Build history of the part. All positions in model axes, mm. A direction names the side the tool comes from. Coordinates: 2 decimals unless noted, no trailing zeros. Write each loop counter-clockwise with the first axis right and the second up, starting at its lowest first coordinate (ties: lowest second). Pieces come first, ordered by that corner, then holes.
from build123d import *

# Parameters (mm, degrees)
SKETCH1_R           = 1.5
BOSS_EXTRUDE1_DEPTH = 2
SKETCH2_W           = 30.25
SKETCH2_H           = 7
BOSS_EXTRUDE2_DEPTH = 10
CUT_EXTRUDE1_DEPTH  = 72.688562547
SKETCH4_W           = 15
SKETCH4_H           = 18.5
BOSS_EXTRUDE3_DEPTH = 15
SKETCH5_W           = 6.5
SKETCH5_H           = 4
BOSS_EXTRUDE4_DEPTH = 4
SKETCH6_R           = 1.5
BOSS_EXTRUDE5_DEPTH = 5
FILLET1_R           = 1.5
FILLET2_R           = 1.5
FILLET3_R           = 1.5
FILLET4_R           = 1.5
FILLET5_R           = 1.5


with BuildPart() as part:
    # Sketch1 → Boss-Extrude1 (new body)
    with BuildSketch(Plane(origin=(0, 0, 0), x_dir=(1, 0, 0), z_dir=(0, 1, 0))):
        with BuildLine():
            Line((-35, -22.5), (35, -22.5))
            ThreePointArc((35, -22.5), (35.707106781, -22.207106781), (36, -21.5))
            Line((36, -21.5), (36, 21.5))
            ThreePointArc((36, 21.5), (35.707106781, 22.207106781), (35, 22.5))
            Line((35, 22.5), (-35, 22.5))
            ThreePointArc((-35, 22.5), (-35.707106781, 22.207106781), (-36, 21.5))
            Line((-36, 21.5), (-36, -21.5))
            ThreePointArc((-36, -21.5), (-35.707106781, -22.207106781), (-35, -22.5))
        make_face()
        with Locations(Location((-33.5, 20, 0), (0, 0, 270))):
            Circle(SKETCH1_R, mode=Mode.SUBTRACT)
        with Locations(Location((33.5, 20, 0), (0, 0, 90))):
            Circle(SKETCH1_R, mode=Mode.SUBTRACT)
        with Locations(Location((33.5, -20, 0), (0, 0, 270))):
            Circle(SKETCH1_R, mode=Mode.SUBTRACT)
        with Locations(Location((-33.5, -20, 0), (0, 0, 90))):
            Circle(SKETCH1_R, mode=Mode.SUBTRACT)
    extrude(amount=BOSS_EXTRUDE1_DEPTH)

    # Sketch2 → Boss-Extrude2 (add)
    with BuildSketch(Plane(origin=(0, 2, 0), x_dir=(1, 0, 0), z_dir=(0, 1, 0))):
        with Locations((-15.875, 16)):
            Rectangle(SKETCH2_W, SKETCH2_H)
        with Locations((15.875, 16)):
            Rectangle(SKETCH2_W, SKETCH2_H)
    extrude(amount=BOSS_EXTRUDE2_DEPTH)

    # Sketch3 → Cut-Extrude1 (cut, through all)
    with BuildSketch(Plane.ZY.offset(31)):
        Polygon((-19.5, 8), (-18.5, 12), (-19.5, 12), align=None)
        Polygon((-12.5, 8), (-14, 12), (-12.5, 12), align=None)
    extrude(amount=-CUT_EXTRUDE1_DEPTH, mode=Mode.SUBTRACT)

    # Sketch4 → Boss-Extrude3 (add)
    with BuildSketch(Plane(origin=(0, 2, 0), x_dir=(1, 0, 0), z_dir=(0, 1, 0))):
        with Locations((26, 2.25)):
            Rectangle(SKETCH4_W, SKETCH4_H)
        with Locations((8.5, 2.25)):
            Rectangle(SKETCH4_W, SKETCH4_H)
        with Locations((-8.5, 2.25)):
            Rectangle(SKETCH4_W, SKETCH4_H)
        with Locations((-26, 2.25)):
            Rectangle(SKETCH4_W, SKETCH4_H)
    extrude(amount=BOSS_EXTRUDE3_DEPTH)

    # Sketch5 → Boss-Extrude4 (add)
    with BuildSketch(Plane(origin=(0, 2, 0), x_dir=(1, 0, 0), z_dir=(0, 1, 0))):
        with Locations((-26, -10.5)):
            Rectangle(SKETCH5_W, SKETCH5_H)
        with Locations((-8.5, -10.5)):
            Rectangle(SKETCH5_W, SKETCH5_H)
        with Locations((8.5, -10.5)):
            Rectangle(SKETCH5_W, SKETCH5_H)
        with Locations((26, -10.5)):
            Rectangle(SKETCH5_W, SKETCH5_H)
    extrude(amount=BOSS_EXTRUDE4_DEPTH)

    # Sketch6 → Boss-Extrude5 (add)
    with BuildSketch(Plane(origin=(0, 2, 0), x_dir=(1, 0, 0), z_dir=(0, 1, 0))):
        with Locations(Location((28, -19, 0), (0, 0, 90))):
            Circle(SKETCH6_R)
        with Locations(Location((21.5, -19, 0), (0, 0, 90))):
            Circle(SKETCH6_R)
        with Locations(Location((15, -19, 0), (0, 0, 90))):
            Circle(SKETCH6_R)
        with Locations(Location((8.5, -19, 0), (0, 0, 90))):
            Circle(SKETCH6_R)
        with Locations(Location((2, -19, 0), (0, 0, 90))):
            Circle(SKETCH6_R)
    extrude(amount=BOSS_EXTRUDE5_DEPTH)

    # Fillet1
    fillet1_edges = [part.edges().sort_by_distance(p)[0] for p in [
        (2, 7, 20.5),
    ]]
    fillet(fillet1_edges, radius=FILLET1_R)

    # Fillet2
    fillet2_edges = [part.edges().sort_by_distance(p)[0] for p in [
        (8.5, 7, 20.5),
    ]]
    fillet(fillet2_edges, radius=FILLET2_R)

    # Fillet3
    fillet3_edges = [part.edges().sort_by_distance(p)[0] for p in [
        (15, 7, 20.5),
    ]]
    fillet(fillet3_edges, radius=FILLET3_R)

    # Fillet4
    fillet4_edges = [part.edges().sort_by_distance(p)[0] for p in [
        (21.5, 7, 20.5),
    ]]
    fillet(fillet4_edges, radius=FILLET4_R)

    # Fillet5
    fillet5_edges = [part.edges().sort_by_distance(p)[0] for p in [
        (28, 7, 20.5),
    ]]
    fillet(fillet5_edges, radius=FILLET5_R)


solid = part.part
(1) Probe L1, parallel to X at y = 2.75, z = -6; L2, parallel to X at y = 0.65, z = 20; L3, parallel to Z at x = 5, y = 4.75. List the from-to ranges inside material, lowest first.
(2) Slice it at A-A, the plane x = 25. List the corners of the cut face in (y, z), and give its area (4 significant figures).
(3) Slice it at C-C, the plane z = -10. List the corners of the cut face in (x, y), and give its area (3 significant figures).
(4) 3-axis set-ups, long thin cutter, end or side, ignore diameter. For faces 4 (the flat face through (26, 9, 7)), 5 (the flat face through (-9, 6, 10)), 6 (the cylindrical face through (14.93, 3.73, 20.5)): which of +Z, -Z, +X, -X, +Y, -Y reach the whole face in a straight line?
(5) Slice it at D-D, the plane y = 4.5. Give the number of separate pieces and of enclosed holes in the cut face, and give its area (3 significant figures).
(6) Slice it at B-B, the plane y = 9. List the corners of the cut face in (x, z) (3 decimals), and give its area (3 significant figures).
(7) Flat gauge pins, fed straight in: P1, Ø6.5, axis at x = -13, y = 6.5, coming from the -Z side; P2, Ø1, axis at x = -28.5, y = 7.5, coming from the +Z side; P3, Ø5, axis at x = -15, z = -17, coming from the +Y side. Where does each tip first touch, or does it go through?
(8) Two-plate mould, pull along X, no slides. Class faces 1 (the flat face through (8, 4, 8.5)), 2 (the flat face through (18.5, 9, -2)), 3 (the flat face through (-33.5, 9, -2)): pulls with the +X half, pulls with the -X half, needs draft (parallel to the pull), parting line crosses it, or undercut.
Results:
1. L1: x = -33.5 to -18.5, -16 to -1, 1 to 16, 18.5 to 33.5
1. L2: x = -36 to -35, -32 to 32, 35 to 36
1. L3: z = -19.5 to -12.5, -11.5 to 7
2. outline: (0, -22.5) - (2, -22.5) - (2, -19.5) - (8, -19.5) - (12, -18.5) - (12, -14) - (8, -12.5) - (2, -12.5) - (2, -11.5) - (17, -11.5) - (17, 7) - (2, 7) - (2, 8.5) - (6, 8.5) - (6, 12.5) - (2, 12.5) - (2, 22.5) - (0, 22.5) - close
2. area: 448.5 mm2
3. outline: (-36, 0) - (36, 0) - (36, 2) - (33.5, 2) - (33.5, 17) - (18.5, 17) - (18.5, 2) - (16, 2) - (16, 17) - (1, 17) - (1, 2) - (-1, 2) - (-1, 17) - (-16, 17) - (-16, 2) - (-18.5, 2) - (-18.5, 17) - (-33.5, 17) - (-33.5, 2) - (-36, 2) - close
3. area: 1,040 mm2
4. face 4: +X, -X, +Y
4. face 5: +Z, +X, -X, +Y
4. face 6: +Y
5. separate pieces: 15
5. enclosed holes: 0
5. area: 1,670 mm2
6. outline: (-33.5, -11.5) - (-18.5, -11.5) - (-18.5, 7) - (-33.5, 7) - close; (-31, -19.25) - (-0.75, -19.25) - (-0.75, -12.875) - (-31, -12.875) - close; (-16, -11.5) - (-1, -11.5) - (-1, 7) - (-16, 7) - close; (0.75, -19.25) - (31, -19.25) - (31, -12.875) - (0.75, -12.875) - close; (1, -11.5) - (16, -11.5) - (16, 7) - (1, 7) - close; (18.5, -11.5) - (33.5, -11.5) - (33.5, 7) - (18.5, 7) - close
6. area: 1,500 mm2
7. P1: stops at z = -19.5
7. P2: stops at z = 7
7. P3: stops at y = 12
8. face 1: needs draft
8. face 2: undercut
8. face 3: pulls with the -X half
